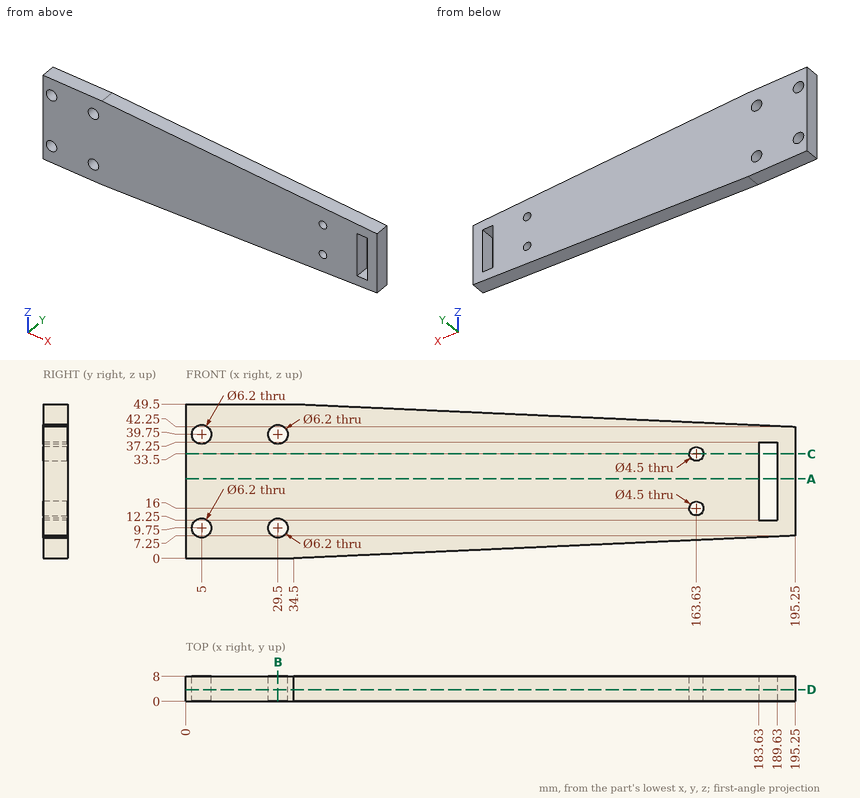
Source: three-view drawing plus pictorial views. Frame: mm from the lowest corner of the part. Round coordinates to 2 decimals unless told otherwise and drop trailing zeros. Order: outer loops, then holes, each group sorted by start corner. A loop starts at its lowest first (then second) coordinate and runs counter-clockwise, first axis right, second up. Notation, with made-up numbers: M 35,51.5 L 55,51.5 A16 ccw 55,59.5 Z; hole C 33.25,47.25 d4. An arc over 180 degrees is marked long. One line per item, written item: value.
(1) Cut plane B-B (x = 29.5). Return the cut outline in (y, z), and give its area (3 significant figures).
Result sheet:
outline: M 0,0 L 8,0 L 8,6.65 L 0,6.65 Z; M 0,12.85 L 8,12.85 L 8,36.65 L 0,36.65 Z; M 0,42.85 L 8,42.85 L 8,49.5 L 0,49.5 Z
area: 297 mm2
(2) Cut plane A-A (z = 25.5). Return the cut outline in (x, y).
Result sheet:
outline: M 0,0 L 183.63,0 L 183.63,8 L 0,8 Z; M 189.63,0 L 195.25,0 L 195.25,8 L 189.63,8 Z
(3) Cut plane D-D (y = 3.75). Return the cut outline in (x, z).
Result sheet:
outline: M 0,0 L 34.5,0 L 195.25,7.25 L 195.25,42.25 L 34.5,49.5 L 0,49.5 Z; hole C 5,9.75 d6.2; hole C 5,39.75 d6.2; hole C 29.5,9.75 d6.2; hole C 29.5,39.75 d6.2; hole C 163.63,16 d4.5; hole C 163.63,33.5 d4.5; hole M 183.63,12.25 L 189.63,12.25 L 189.63,37.25 L 183.63,37.25 Z
(4) Line query: probe 1 along X at (y, z) = (3.75, 16); probe 2 along X at (y, z) = (2, 39.75); probe 3 along X at (y, z) = (5, 28). Output: solid intervals per line, ascending. Write a range as [from, to].
Result sheet:
probe 1: [0, 161.38], [165.88, 183.63], [189.63, 195.25]
probe 2: [0, 1.9], [8.1, 26.4], [32.6, 195.25]
probe 3: [0, 183.63], [189.63, 195.25]
(5) Pin query (flat end, axial travel): P1, Ø1, axis at x = 100.5, y = 4.5, coming from the +Z side; P2, Ø2, axis at x = 48.5, y = 7, coming from the -Z side; P3, Ø1.8, axis at x = 186.5, y = 2.5, coming from the +Z side; P4, Ø1.5, axis at y = 4, z = 24, coming from the -X side. Return the tip coordinate at first contact, or that it passes through.
Result sheet:
P1: z = 46.55
P2: z = 0.59
P3: z = 42.69
P4: x = 0
(6) Cut plane C-C (z = 33.5). Return the cut outline in (x, y), and give its area (3 significant figures).
Result sheet:
outline: M 0,0 L 161.38,0 L 161.38,8 L 0,8 Z; M 165.88,0 L 183.63,0 L 183.63,8 L 165.88,8 Z; M 189.63,0 L 195.25,0 L 195.25,8 L 189.63,8 Z
area: 1,480 mm2
